Autodesk Inventor part; units mm, degrees
ref_plane "YZ Plane" through (0, 0, 0) normal (1, 0, 0) x (0, 1, 0)
ref_plane "XZ Plane" through (0, 0, 0) normal (0, 1, 0) x (-1, 0, 0)
ref_plane "XY Plane" through (0, 0, 0) normal (0, 0, 1) x (1, 0, 0)
sketch "Sketch1" plane through (0, 0, 0) normal (0, 1, 0) x (-1, 0, 0)
  line L0 (14.2949, 30.3382) -> (-112.7051, 30.3382)
  line L1 (-112.7051, 30.3382) -> (-112.7051, -20.4618)
  line L2 (-112.7051, -20.4618) -> (14.2949, -20.4618)
  line L3 (14.2949, -20.4618) -> (14.2949, 30.3382)
  point P0 (0, 0)
  dimension "d0" = 127
  dimension "d1" = 50.8
extrude "Extrusion1" add sketch "Sketch1" along normal blind 76.2
sketch "Sketch2" plane through (0, 76.2, 0) normal (0, 1, 0) x (1, 0, 0)
  line L0 (-14.2949, 20.4618) -> (-14.2949, -30.3382)
  line L1 (-14.2949, -4.9382) -> (4.7551, -4.9382)
  line L2 (4.7551, -4.9382) -> (30.1551, -4.9382)
  line L3 (30.1551, -4.9382) -> (61.9051, -4.9382)
  line L4 (61.9051, -4.9382) -> (93.6551, -4.9382)
  point P0 (0, 0)
  dimension "d4" = 19.05
  dimension "d5" = 25.4
  dimension "d6" = 31.75
  dimension "d7" = 31.75
hole "Hole1" at (93.6551, 76.2, 4.9382) direction (0, -1, 0) diameter 6.35 depth 25.4 tip angle 118
hole "Hole2" at (93.6551, 76.2, 4.9382) direction (0, -1, 0) diameter 9.525 depth 6.35 tip angle 118
hole "Hole3" at (61.9051, 76.2, 4.9382) direction (0, -1, 0) diameter 12.7 depth 0.508 tip angle 118
hole "Hole4" at (30.1551, 76.2, 4.9382) direction (0, -1, 0) diameter 12.7 depth 76.2 tip angle 118 countersink diameter 25.4 countersink angle 82
hole "Hole5" at (4.7551, 76.2, 4.9382) direction (0, -1, 0) diameter 12.7 depth 76.2 tip angle 118 counterbore diameter 19.05 counterbore depth 6.35
properties part number "7.2 part 4"
Verification items for the finished model (mm, model axes). A direction names the side the tool comes from. Round coordinates to 2 decimals unless told otherwise and drop trailing zeros. Order: outer loops, then holes, each group sorted by start corner. A loop starts at its lowest first (then second) coordinate and runs counter-clockwise, first axis right, second up.
1. Release check for a two-part mould opening along Z. For faces 3 (the flat face through (50, 0, 5)), 4 (the cylindrical face through (14.054, 72.981, 2.873)), 5 (the flat face through (48, 38, 30.338)) record: +Z half, -Z half, draft (parallel to the pull), parting line (faces both ways), or undercut.
Final values:
face 3: draft
face 4: undercut
face 5: +Z half
2. Access from +Z, -Z, +X, -X, +Y, -Y to the whole of each face (thin tool, end or side, straight path). Record for faces 1 (the flat face through (50, 38, -20.462)), 2 (the cylindrical face through (55.61, 75.94, 4.11)).
Final values:
face 1: -Z, +X, -X, +Y, -Y
face 2: +Y
3. Section check A-A on y = 57.5. Record the cut outline in (x, z) (3 decimals).
Final values:
outline: (-14.295, -20.462) - (112.705, -20.462) - (112.705, 30.338) - (-14.295, 30.338) - close; hole circle Ø12.7 at (4.755, 4.938); hole circle Ø12.7 at (30.155, 4.938); hole circle Ø6.35 at (93.655, 4.938)
4. Go/stop test with a flat-tipped pin: P1, Ø7.5, axis at x = 4.76, z = 4.94, coming from the -Y side. Record where the tip stops, or that it passes through.
Final values:
P1: passes through
5. Section check B-B on y = 40.5. Record the cut outline in (x, z), then the cut area to 3 significant figures.
Final values:
outline: (-14.29, -20.46) - (112.71, -20.46) - (112.71, 30.34) - (-14.29, 30.34) - close; hole circle Ø12.7 at (4.76, 4.94); hole circle Ø12.7 at (30.16, 4.94)
area: 6,200 mm2
6. Thickness scan on L1, parallel to X at y = 73.5, z = 1.5; L2, parallel to Z at x = 30, y = 55; L3, parallel to Z at x = 13, y = 71. Record the ranges inside material, lowest first.
Final values:
L1: x = -14.29 to -4.13, 13.64 to 20.39, 39.92 to 90.36, 96.95 to 112.71
L2: z = -20.46 to -1.41, 11.29 to 30.34
L3: z = -20.46 to 0.17, 9.71 to 30.34
